Model file for the job. Use its own axes, mm. Face numbers are marked on the shaded views. Round coordinates to 2 decimals unless told otherwise and drop trailing zeros. Loops run counter-clockwise (first coordinate to the right, second up) from the corner with the lowest first, then second, coordinate; pieces in that order, holes last.
from build123d import *

# Parameters (mm, degrees)
SKETCH_1_R          = 1.55
EXTRUDE_1_DEPTH     = 2
FILLET_1_R          = 3
FILLET_2_R          = 0.2
SKETCH_3_R          = 0.75
CUT_EXTRUDE_1_DEPTH = 1


with BuildPart() as part:
    # 草图1 → 凸台-拉伸1 (new body)
    with BuildSketch(Plane(origin=(0, 0, 0), x_dir=(1, 0, 0), z_dir=(0, 1, 0))):
        with BuildLine():
            Line((-9.427629845, 12.118007633), (-14.205972572, 5.57250637))
            ThreePointArc((-14.205972572, 5.57250637), (-13.333741258, -0.01669863), (-7.744536258, 0.855532684))
            Line((-7.744536258, 0.855532684), (-2.966193531, 7.401033946))
            ThreePointArc((-2.966193531, 7.401033946), (2.156455687, 5.844533995), (7.508476858, 5.702771934))
            Line((7.508476858, 5.702771934), (9.973957748, -2.017173013))
            ThreePointArc((9.973957748, -2.017173013), (15.001264118, -4.610663069), (17.594754173, 0.416643301))
            Line((17.594754173, 0.416643301), (15.129273283, 8.136588247))
            Line((15.129273283, 8.136588247), (19.53886034, 20.548398832))
            ThreePointArc((19.53886034, 20.548398832), (2.94865648, 10.730730666), (-9.689752685, 25.287244194))
            Line((-9.689752685, 25.287244194), (-9.427629845, 12.118007633))
        make_face()
        with Locations(Location((13.784355961, -0.800264856, 0), (0, 0, 270))):
            Circle(SKETCH_1_R, mode=Mode.SUBTRACT)
        with Locations(Location((-10.975254415, 3.214019527, 0), (0, 0, 270))):
            Circle(SKETCH_1_R, mode=Mode.SUBTRACT)
    extrude(amount=EXTRUDE_1_DEPTH)

    # 圆角1
    fillet_1_edges = [part.edges().sort_by_distance(p)[0] for p in [
        (-9.427629845, 1, -12.118007633),
        (15.129273283, 1, -8.136588247),
        (7.508476858, 1, -5.702771934),
        (-2.966193531, 1, -7.401033946),
    ]]
    fillet(fillet_1_edges, radius=FILLET_1_R)

    # 草图2 → 切除-旋转1 (revolve, cut)
    with BuildSketch(Plane(origin=(5.357266973, 0, 0), x_dir=(0, -1, 0), z_dir=(-1, 0, 0))):
        with BuildLine():
            Line((43.030031962, -25.586742765), (-7.030031962, -25.586742765))
            ThreePointArc((-7.030031962, -25.586742765), (18, -0.556710804), (43.030031962, -25.586742765))
        make_face()
    revolve(axis=Axis((5.357266973, -43.030031962, -25.586742765), (0, 1, 0)), mode=Mode.SUBTRACT)

    # 圆角2
    # the kernel refuses this fillet: 0.2 mm, written as the material it takes off along each edge
    with BuildSketch(Plane(origin=(19.53886034, -18, -20.548398832), x_dir=(-0.1606859623720409, 0.8772773226728997, 0.4522880947144644), z_dir=(-0.29368936055859224, -0.47998385298244073, 0.8266571601158587))) as fillet_2_piece_1:
        with BuildLine():
            CenterArc((20.396862817, 0.2), FILLET_2_R, 143.943391902, 126.056608098)
            Line((20.396862817, 0), (20, 0))
            ThreePointArc((20, 0), (20.118215024, 0.158394169), (20.235175643, 0.317716854))
        make_face()
    revolve(axis=Axis((19.53886034, -18, -20.548398832), (-0.9422985625539585, 0, -0.3347736832678813)), revolution_arc=31.526759785, mode=Mode.SUBTRACT)
    with BuildSketch(Plane(origin=(-9.689752685, -18, -25.287244194), x_dir=(-0.0009868358148414909, 0.9987697013737694, -0.049579328079614966), z_dir=(-0.01987575403412073, -0.049589148185379746, -0.9985719156794987))) as fillet_2_piece_2:
        with BuildLine():
            CenterArc((20.396862817, 0.2), FILLET_2_R, 143.943391902, 126.056608098)
            ThreePointArc((20.235175643, 0.317716854), (20.118215024, 0.158394169), (20, 0))
            Line((20, 0), (20.396862817, 0))
        make_face()
    revolve(axis=Axis((-9.689752685, -18, -25.287244194), (0.9998019706705172, 0, -0.019900237268694068)), revolution_arc=31.526762102, mode=Mode.SUBTRACT)

    # 草图3 → 切除-拉伸1 (cut)
    with BuildSketch(Plane(origin=(0, 2, 0), x_dir=(1, 0, 0), z_dir=(0, 1, 0))):
        with Locations(Location((-8.027145861, 7.252417223, 0), (0, 0, 270))):
            Circle(SKETCH_3_R)
    extrude(amount=-CUT_EXTRUDE_1_DEPTH, mode=Mode.SUBTRACT)


solid = part.part
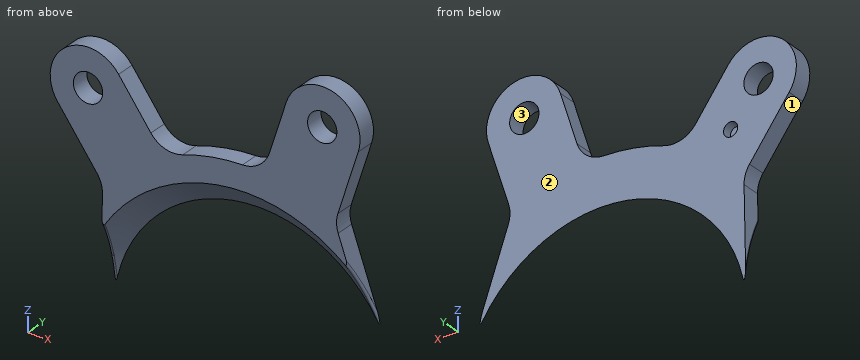
Q1. Probe line 1 (X direction, y = 1.2, z = -4.25); line 2 (X direction, y = 1.65, z = -2.5); line 3 (Z direction, x = -12, y = 1.65). List the from-to ranges inside material, lowest first.
Q2. Pull direction Z, two halves, no side cores. Call the marked faces 1, 2 and 3: pulls with the +Z half, pulls with the -Z half, needs draft (parallel to the pull), parting line crosses it, or undercut.
Q3. Flat gauge pin, fed straight in: P1, Ø0.8, axis at x = -8, z = -7, coming from the +Y side. Where does the tip first touch, or does it go through?
Q4. Slice it at D-D on x = 9.5. Give the cut face in (y, z), plus the area to 3 significant figures.
Q5. Slice it at A-A on x = -10.5. Give the cut face in (y, z).
Q6. Slice it at C-C on y = 1.35. State how many separate pieces and enclosed holes the cut face has, plus the area to 3 significant figures.
Q7. Slice it at B-B on z = -2.5. Give the cut face in (x, y), plus the area to 3 significant figures.
Reply:
1. line 1: x = -14.84 to -12.13, -9.82 to -5.27, 7.85 to 16.37
1. line 2: x = -14.91 to -12.35, -9.6 to -6.54, 8.53 to 16.93
1. line 3: z = -8.59 to -4.38, -2.05 to 0.65
2. face 1: pulls with the -Z half
2. face 2: needs draft
2. face 3: undercut
3. P1: stops at y = 1
4. outline: (0, -8.69) arc R24.68 cw to (2, -11.12) - (2, 0.53) - (0, 0.53) - close
4. area: 20.8 mm2
5. outline: (0, -10.65) - (2, -10.65) - (2, -4.69) - (0, -4.69) - close; (0, -1.74) - (2, -1.74) - (2, 0.76) - (0, 0.76) - close
6. separate pieces: 1
6. enclosed holes: 3
6. area: 283 mm2
7. outline: (-14.91, 0) - (-12.35, 0) - (-12.35, 2) - (-14.91, 2) - close; (-9.6, 0) - (-6.54, 0) - (-6.54, 2) - (-9.6, 2) - close; (8.53, 0) - (16.93, 0) - (16.93, 2) - (8.53, 2) - close
7. area: 28.0 mm2
